Check sheet for the modelled part. Datum: model origin and axes. Units: mm. Face numbers are marked on the shaded views. A direction names the side the tool comes from. Give positions to 0.01 mm unless a question says otherwise; leave off trailing zeros. Order: outer loops, then holes, each group sorted by start corner. A loop starts at its lowest first (then second) coordinate and runs counter-clockwise, first axis right, second up.
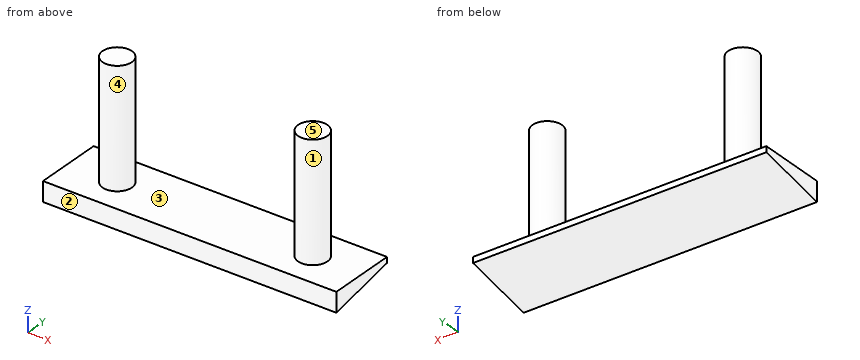
```python
from build123d import *

# Parameters (mm, degrees)
F0_W     = 38.1
F0_H     = 8.89
F1_DEPTH = 2.54
F2_R     = 1.905
F3_DEPTH = 15.24
F5_DEPTH = 38.1


with BuildPart() as f1:
    # F0 (on Top) → F1 (new body)
    with BuildSketch(Plane.XY):
        with Locations((19.05, 4.445)):
            Rectangle(F0_W, F0_H)
    extrude(amount=F1_DEPTH)

    # F2 (on face) → F3 (join)
    with BuildSketch(Plane.XY.offset(2.54)):
        with Locations((6.35, 4.445)):
            Circle(F2_R)
        with Locations((31.75, 4.445)):
            Circle(F2_R)
    extrude(amount=F3_DEPTH)

    # F4 (on face) → F5 (cut)
    with BuildSketch(Plane.YZ.offset(38.1)):
        Polygon((8.89, 0), (8.89, 1.798025), (0, 0), align=None)
    extrude(amount=-F5_DEPTH, mode=Mode.SUBTRACT)


solid = f1.part
```
(1) Sectioned sample at A-A (x = 6.35). Enter the section's corners in (y, z).
(2) Release check for a two-part mould opening along X. For the marked faces 1, 2 and 3 record: released by +X, released by -X, zero draft, split by the parting line, or undercut.
(3) Thickness scan on L1, parallel to X at y = 4.5, z = 10; L2, parallel to X at y = 3.5, z = 10; L3, parallel to Z at x = 15, y = 2.75. Record the ranges inside material, lowest first.
(4) Sectioned sample at D-D (x = 31). Enter the section's corners in (y, z), plus the area to 3 significant figures.
(5) Sectioned sample at B-B (z = 16.75). Enter the section's corners in (x, y) (3 decimals).
(6) Sectioned sample at C-C (y = 7.5). Enter the section's corners in (x, z), plus the area to 3 significant figures.
(7) Go/stop test with flat-tipped pins: P1, Ø5, axis at y = 4, z = 3.5, coming from the +X side; P2, Ø1, axis at x = 26, y = 4.5, coming from the +Z side; P3, Ø2, axis at y = 7.5, z = 10, coming from the -X side; P4, Ø8, axis at x = 33.5, z = 14, coming from the +Y side. Record where each tip stops, or that it passes through.
(8) Tool access check on the marked faces 4 and 5. Record the directions out of +Z, -Z, +X, -X, +Y, -Y that give a thin tool (end or side, any length) a straight path to the whole face; none if there is none.
Values follow:
1. outline: (0, 0) - (8.89, 1.8) - (8.89, 2.54) - (6.35, 2.54) - (6.35, 17.78) - (2.54, 17.78) - (2.54, 2.54) - (0, 2.54) - close
2. face 1: undercut
2. face 2: zero draft
2. face 3: undercut
3. L1: x = 4.45 to 8.25, 29.85 to 33.65
3. L2: x = 4.7 to 8, 30.1 to 33.4
3. L3: z = 0.56 to 2.54
4. outline: (0, 0) - (8.89, 1.8) - (8.89, 2.54) - (6.2, 2.54) - (6.2, 17.78) - (2.69, 17.78) - (2.69, 2.54) - (0, 2.54) - close
4. area: 68.0 mm2
5. outline: circle Ø3.81 at (6.35, 4.445); circle Ø3.81 at (31.75, 4.445)
6. outline: (0, 1.52) - (38.1, 1.52) - (38.1, 2.54) - (0, 2.54) - close
6. area: 39.0 mm2
7. P1: stops at x = 38.1
7. P2: stops at z = 2.54
7. P3: passes through
7. P4: stops at y = 6.35
8. face 4: +Z
8. face 5: +Z, +X, -X, +Y, -Y
